The listing builds one solid part. Answer for the finished solid, in the listing's coordinates (mm). Round coordinates to 2 decimals unless told otherwise and drop trailing zeros. Write each loop counter-clockwise with the first axis right and the second up, starting at its lowest first coordinate (ties: lowest second). Pieces come first, ordered by that corner, then holes. Notation, with made-up numbers: M 67,-30.5 L 91,-30.5 A5 cw 91,-23.5 Z; hole C -13.75,-39 d11. An arc over 180 degrees is marked long. One line per item, written item: value. Start each with the question number.
(1) Section B-B (x = 20.32) is taken. Determine the outline of the cut face in (y, z) (3 decimals), plus the area to 3 significant figures.
(2) Consider probe 1 along X at (y, z) = (0, -1.5); probe 2 along X at (y, z) = (-10, -4.25); probe 3 along X at (y, z) = (20, -6.25). Determine where each line is inside the solid, lowest interval first.
(3) Section D-D (x = 0) is taken. Determine the outline of the cut face in (y, z).
(4) Section A-A (z = -5.08) is taken. Determine the outline of the cut face in (x, y) (3 decimals), plus the area to 3 significant figures.
(5) Given P1, Ø3.5, axis at x = 30.5, y = 1, coming from the +Z side; P2, Ø5, axis at x = -20.32, z = -5.08, coming from the -Y side, each flat-ended and moving along its own axis, determine where each tip first touches the part or whether it passes through.
(6) Section C-C (y = 0) is taken. Determine the outline of the cut face in (x, z) (3 decimals), plus the area to 3 significant figures.
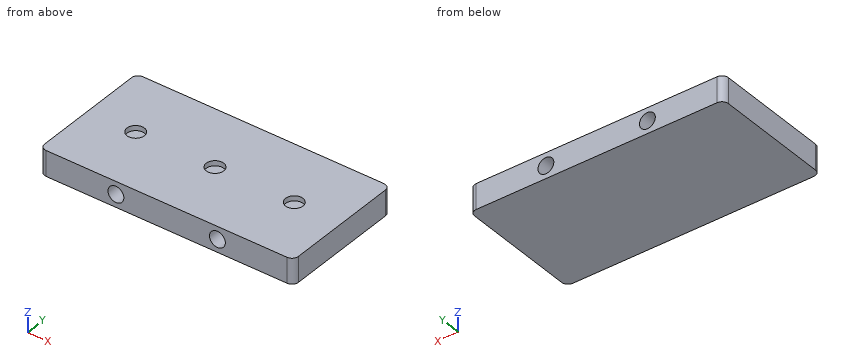
Autodesk Fusion 360 part; units mm, degrees
sketch "Sketch1" plane through (0, 0, 0) normal (0, 0, 1) x (1, 0, 0)
  line L0 (50.8, -25.4) -> (-50.8, -25.4)
  line L1 (-50.8, -25.4) -> (-50.8, 25.4)
  line L2 (-50.8, 25.4) -> (50.8, 25.4)
  line L3 (50.8, 25.4) -> (50.8, -25.4)
  line L4 (50.8, -25.4) -> (-50.8, 25.4) construction
  line L5 (-50.8, -25.4) -> (50.8, 25.4) construction
  dimension "d2" = 101.6
  dimension "d8" = 50.8
extrude "Extrude1" add sketch "Sketch1" against normal blind 10.16
sketch "Sketch2" plane through (0, 0, 0) normal (0, 0, 1) x (-1, 0, 0)
  line L0 (-50.8, -25.4) -> (50.8, -25.4)
  line L1 (50.8, -25.4) -> (50.8, 25.4)
  line L2 (50.8, 25.4) -> (-50.8, 25.4)
  line L3 (-50.8, 25.4) -> (-50.8, -25.4)
  circle A0 centre (31.75, 0) radius 3.5
  circle A1 centre (0, 0) radius 3.5
  circle A2 centre (-31.75, 0) radius 3.5
  line L4 (12.7, -25.4) -> (12.7, 25.4) construction
  dimension "d11" = 7
  dimension "d12" = 19.05
  dimension "d13" = 7
  dimension "d14" = 50.8
  dimension "d15" = 7
  dimension "d16" = 19.05
  dimension "d17" = 25.4
  dimension "d18" = 25.4
  dimension "d19" = 25.4
  dimension "d22" = 38.1
extrude "Extrude2" cut sketch "Sketch2" against normal blind 2 contours A0 | A1 | A2
sketch "Sketch3" plane through (0, -25.4, 0) normal (0, -1, 0) x (1, 0, 0)
  line L0 (50.8, 0) -> (-50.8, 0)
  line L1 (-50.8, 0) -> (-50.8, -10.16)
  line L2 (-50.8, -10.16) -> (50.8, -10.16)
  line L3 (50.8, -10.16) -> (50.8, 0)
  circle A0 centre (-20.32, -5.08) radius 3.175
  circle A1 centre (20.32, -5.08) radius 3.175
  dimension "d23" = 30.48
  dimension "d24" = 30.48
  dimension "d25" = 6.35
  dimension "d26" = 6.35
  dimension "d27" = 5.08
  dimension "d28" = 5.08
extrude "Extrude3" cut sketch "Sketch3" against normal through all contours A0 | A1
fillet "Fillet1" radius 2.54 4 edges at (-50.8, -25.4, -5.08) (-50.8, 25.4, -5.08) (50.8, -25.4, -5.08) (50.8, 25.4, -5.08)
Recorded:
1. outline: M -25.4,-10.16 L 25.4,-10.16 L 25.4,-8.255 L -25.4,-8.255 Z; M -25.4,-1.905 L 25.4,-1.905 L 25.4,0 L -25.4,0 Z
1. area: 194 mm2
2. probe 1: x = -50.8 to -35.25, -28.25 to -3.5, 3.5 to 28.25, 35.25 to 50.8
2. probe 2: x = -50.8 to -23.38, -17.26 to 17.26, 23.38 to 50.8
2. probe 3: x = -50.8 to -23.27, -17.37 to 17.37, 23.27 to 50.8
3. outline: M -25.4,-10.16 L 25.4,-10.16 L 25.4,0 L 3.5,0 L 3.5,-2 L -3.5,-2 L -3.5,0 L -25.4,0 Z
4. outline: M -50.8,-22.86 A2.54 ccw -48.26,-25.4 L -23.495,-25.4 L -23.495,25.4 L -48.26,25.4 A2.54 ccw -50.8,22.86 Z; M -17.145,-25.4 L 17.145,-25.4 L 17.145,25.4 L -17.145,25.4 Z; M 23.495,-25.4 L 48.26,-25.4 A2.54 ccw 50.8,-22.86 L 50.8,22.86 A2.54 ccw 48.26,25.4 L 23.495,25.4 Z
4. area: 4,510 mm2
5. P1: stops at z = -2
5. P2: passes through
6. outline: M -50.8,-10.16 L 50.8,-10.16 L 50.8,0 L 35.25,0 L 35.25,-2 L 28.25,-2 L 28.25,0 L 3.5,0 L 3.5,-2 L -3.5,-2 L -3.5,0 L -28.25,0 L -28.25,-2 L -35.25,-2 L -35.25,0 L -50.8,0 Z; hole C -20.32,-5.08 d6.35; hole C 20.32,-5.08 d6.35
6. area: 927 mm2
